Could you check a few things on this model? Use its own coordinates, in mm. A direction names the side the tool comes from. Coordinates: 2 decimals unless noted, no trailing zeros. Loops run counter-clockwise (first coordinate to the right, second up) from the corner with the lowest first, then second, coordinate; pieces in that order, holes last. Notation, with made-up numbers: (23.25, -33) - (57.25, -33) arc R28 cw to (57.25, -11) - close; hole circle Ø3 at (72.25, -12.75). An arc over 180 degrees is marked (long way). One line per question, with ' | ' between items. Start each with the question number.
1. I want a section at C-C, the plane y = 5. Write out the boundary of the cut face in (x, z) (3 decimals).
2. I want a section at A-A, the plane y = 40. Write out the boundary of the cut face in (x, z) (3 decimals), then the cut area to 3 significant figures.
3. I'm going to push flat-ended pins straight in: P1, Ø2, axis at y = 11.5, z = 18.5, coming from the -X side; P2, Ø10, axis at y = 5, z = 14, coming from the +X side; P3, Ø0.5, axis at x = 47.5, z = -1.5, coming from the +Y side (3 decimals); P4, Ø7.5, axis at y = 40, z = 14, coming from the -X side. Where does each tip first touch, or does it pass through?
4. I want a section at B-B, the plane z = 14. Write out the boundary of the cut face in (x, y), then the cut area to 3 significant figures.
5. Which directions (+Z, -Z, +X, -X, +Y, -Y) give clear straight access to the entire face, cutting with the end or side of a thin tool? Please do faces 1 (the flat face through (24, 6.125, -4)), 2 (the flat face through (50, 5, -4)), 3 (the flat face through (25, 4, -8)), 4 (the flat face through (38, 6.125, -2)).
6. We'd pull the mould along X, two halves only. Please class faces 5 (the flat face through (0, 3, -4)), 6 (the flat face through (28, 6.125, -4)), 7 (the flat face through (9, 6.125, -4)), 8 (the flat face through (17, 4, 0)): pulls with the +X half, pulls with the -X half, needs draft (parallel to the pull), parting line crosses it, or undercut.
7. I want a section at D-D, the plane z = 1. Write out the boundary of the cut face in (x, y) (1 decimal), then the cut area to 3 significant figures.
8. Please list where these lines run through material, in increasing order: L1, parallel to Y at x = 41, z = 14; L2, parallel to Z at x = 37, y = 40; L3, parallel to Y at x = 26, z = -0.5. Write a range as [from, to].
from build123d import *

# Parameters (mm, degrees)
BLANKSKE_W          = 50
BLANKSKE_H          = 9.5
BLANK_DEPTH         = 8
TOOTHCUTILL_DEPTH   = 52.519413817
TOOTHCUTSIM_DEPTH   = 52.519413817
TEETHCUTS_COUNT     = 11
TEETHCUTS_PITCH     = 4.712388975
BOSS_EXTRUDE8_DEPTH = 45
CUT_EXTRUDE5_DEPTH  = 3
SKETCH20_R          = 4.25
CUT_EXTRUDE6_DEPTH  = 25


with BuildPart() as part:
    # BlankSke → Blank (new body)
    with BuildSketch(Plane.XY):
        with Locations((25, 4.75)):
            Rectangle(BLANKSKE_W, BLANKSKE_H)
    extrude(amount=-BLANK_DEPTH)

    # TooCutSkeIll → ToothCutIll (cut, through all)
    with BuildSketch(Plane.XY):
        with BuildLine():
            Line((-1.713391726, 9.4550228), (-0.92508248, 6.406857118))
            ThreePointArc((-0.92508248, 6.406857118), (-0.791252665, 6.20370072), (-0.561058967, 6.125))
            Line((-0.561058967, 6.125), (0.561058967, 6.125))
            ThreePointArc((0.561058967, 6.125), (0.791252665, 6.20370072), (0.92508248, 6.406857118))
            Line((0.92508248, 6.406857118), (1.713391726, 9.4550228))
            ThreePointArc((1.713391726, 9.4550228), (1.734747547, 9.487441374), (1.771480584, 9.5))
            Line((1.771480584, 9.5), (1.771480584, 9.5254))
            Line((1.771480584, 9.5254), (-1.771480584, 9.5254))
            Line((-1.771480584, 9.5254), (-1.771480584, 9.5))
            ThreePointArc((-1.771480584, 9.5), (-1.734747547, 9.487441374), (-1.713391726, 9.4550228))
        make_face()
    toothcutill = extrude(amount=-TOOTHCUTILL_DEPTH, mode=Mode.SUBTRACT)

    # TooCutSkeSim → ToothCutSim (cut, through all)
    with BuildSketch(Plane.XY):
        Polygon((0.852189273, 6.125), (-0.852189273, 6.125), (-1.731592507, 9.5254), (1.731592507, 9.5254), align=None)
    toothcutsim = extrude(amount=-TOOTHCUTSIM_DEPTH, mode=Mode.SUBTRACT)

    # TeethCuts: ToothCutIll, ToothCutSim ×11
    with Locations(*[(i * TEETHCUTS_PITCH, 0, 0) for i in range(1, TEETHCUTS_COUNT)]):
        add(toothcutill, mode=Mode.SUBTRACT)
        add(toothcutsim, mode=Mode.SUBTRACT)

    # Sketch16 → Boss-Extrude8 (add)
    with BuildSketch(Plane.XZ):
        Polygon((50, 0), (33.849, 0), (33.849, 35), (41.925, 35), align=None)
    extrude(amount=-BOSS_EXTRUDE8_DEPTH)

    # Sketch17 → Cut-Extrude5 (cut)
    with BuildSketch(Plane(origin=(0, 0, 0), x_dir=(-1, 0, 0), z_dir=(0, 0, -1))):
        Polygon((-50, 9.5), (-48.837281476, 9.4550228), (-47.976079023, 6.125), (-46.271700477, 6.125), (-45.410498024, 9.4550228), (-44.124892501, 9.4550228), (-43.263690048, 6.125), (-41.559311502, 6.125), (-40.698109049, 9.4550228), (-39.412503526, 9.4550228), (-38.551301073, 6.125), (-36.846922527, 6.125), (-35.985720074, 9.4550228), (-34.700114551, 9.4550228), (-33.838912098, 6.125), (-33.849, 45), (-50, 45), align=None)
    extrude(amount=-CUT_EXTRUDE5_DEPTH, mode=Mode.SUBTRACT)

    # Sketch20 → Cut-Extrude6 (cut)
    with BuildSketch(Plane.ZY.offset(-33.849)):
        with Locations((14, 40)):
            Circle(SKETCH20_R)
        with Locations((14, 5)):
            Circle(SKETCH20_R)
    extrude(amount=-CUT_EXTRUDE6_DEPTH, mode=Mode.SUBTRACT)


solid = part.part
Results are:
1) outline: (0, -8) - (50, -8) - (50, 0) - (47.751, 9.75) - (33.849, 9.75) - (33.849, 0) - (0, 0) - close; (33.849, 18.25) - (45.789, 18.25) - (41.925, 35) - (33.849, 35) - close
2) outline: (33.849, 3) - (49.308, 3) - (47.751, 9.75) - (33.849, 9.75) - close; (33.849, 18.25) - (45.789, 18.25) - (41.925, 35) - (33.849, 35) - close | area: 267 mm2
3) P1: stops at x = 33.85 | P2: stops at x = 47.92 | P3: stops at y = 6.125 | P4: passes through
4) outline: (33.85, 0) - (46.77, 0) - (46.77, 0.75) - (33.85, 0.75) - close; (33.85, 9.25) - (46.77, 9.25) - (46.77, 35.75) - (33.85, 35.75) - close; (33.85, 44.25) - (46.77, 44.25) - (46.77, 45) - (33.85, 45) - close | area: 362 mm2
5) face 1: +Z, -Z, +Y | face 2: +Z, -Z, +X, +Y, -Y | face 3: -Z, +X, -X, +Y, -Y | face 4: -Z, +Y
6) face 5: pulls with the -X half | face 6: undercut | face 7: undercut | face 8: needs draft
7) outline: (33.8, 0) - (49.8, 0) - (49.8, 9.5) - (48.8, 9.5) - (48, 6.1) - (46.3, 6.1) - (45.4, 9.5) - (44.1, 9.5) - (43.3, 6.1) - (41.6, 6.1) - (40.7, 9.5) - (39.4, 9.5) - (38.6, 6.1) - (36.8, 6.1) - (36, 9.5) - (34.7, 9.5) - (33.8, 6.2) - close | area: 124 mm2
8) L1: y = [0, 0.75], [9.25, 35.75], [44.25, 45] | L2: z = [3, 9.75], [18.25, 35] | L3: y = [0, 9.5]
